Build history of the part. All positions in model axes, mm. A direction names the side the tool comes from. Give positions to 0.01 mm unless a question says otherwise; leave off trailing zeros. Loops run counter-clockwise (first coordinate to the right, second up) from the corner with the lowest first, then second, coordinate; pieces in that order, holes last. Notation, with made-up numbers: (8, 82) - (44, 82) arc R17 cw to (44, 88) - close; hole circle Ø9 at (5.25, 12.5). An arc over 180 degrees is marked (long way). Return JSON: item names as keys, results as strings. Group by question number.
1) Slice it at B-B (y = 46). List the corners of the cut face in (x, z), and give its area (3 significant figures).
2) Mould opens along Y. For faces 3 (the face through (-29.464, 25, 3)), 4 (the face through (-26, 47, 3.556)), 5 (the face through (-40.132, 25, 3)) say: released by +Y, released by -Y, zero draft, split by the parting line, or undercut.
3) Drill centre lines: probe 1 along X at (y, z) = (10.5, 2.6); probe 2 along Y at (x, z) = (-45, 2.8); probe 3 along X at (y, z) = (3.81, 2.65). Where is each one in solid material? Low to high. Write a range as from..to.
4) 3-axis set-ups, long thin cutter, end or side, ignore diameter. For faces 1 (the face through (-50.8, 25, 2)), 2 (the face through (-30.988, 25, 3)): which of +Z, -Z, +X, -X, +Y, -Y reach the whole face in a straight line?
5) Slice it at A-A (z = 2.7). Count the separate pieces of the cut face and the enclosed holes in it, and give its area (3 significant figures).
```python
from build123d import *

# Parameters (mm, degrees)
F0_W     = 50.8
F0_H     = 50.8
F1_DEPTH = 1.524
F2_W     = 50.8
F2_H     = 50.8
F2_W_2   = 46.736
F2_H_2   = 46.736
F2_W_3   = 43.688
F2_H_3   = 43.688
F2_W_4   = 39.624
F2_H_4   = 39.624
F2_W_5   = 36.576
F2_H_5   = 36.576
F2_W_6   = 32.512
F2_H_6   = 32.512
F2_W_7   = 29.464
F2_H_7   = 29.464
F2_W_8   = 25.4
F2_H_8   = 25.4
F2_W_9   = 22.352
F2_H_9   = 22.352
F2_W_10  = 18.288
F2_H_10  = 18.288
F2_W_11  = 15.24
F2_H_11  = 15.24
F2_W_12  = 11.176
F2_H_12  = 11.176
F2_W_13  = 8.128
F2_H_13  = 8.128
F3_DEPTH = 2.032
F4_R     = 1.4605
F5_DEPTH = 25.4


with BuildPart() as f1:
    # F0 (on Top) → F1 (new body)
    with BuildSketch(Plane.XY):
        with Locations((-25.4, 25.4)):
            Rectangle(F0_W, F0_H)
    extrude(amount=F1_DEPTH)

    # F2 (on face) → F3 (join)
    with BuildSketch(Plane.XY.offset(1.524)):
        with Locations((-25.4, 25.4)):
            Rectangle(F2_W, F2_H)
        with Locations((-25.4, 25.4)):
            Rectangle(F2_W_2, F2_H_2, mode=Mode.SUBTRACT)
        with Locations((-25.4, 25.4)):
            Rectangle(F2_W_3, F2_H_3)
        with Locations((-25.4, 25.4)):
            Rectangle(F2_W_4, F2_H_4, mode=Mode.SUBTRACT)
        with Locations((-25.4, 25.4)):
            Rectangle(F2_W_5, F2_H_5)
        with Locations((-25.4, 25.4)):
            Rectangle(F2_W_6, F2_H_6, mode=Mode.SUBTRACT)
        with Locations((-25.4, 25.4)):
            Rectangle(F2_W_7, F2_H_7)
        with Locations((-25.4, 25.4)):
            Rectangle(F2_W_8, F2_H_8, mode=Mode.SUBTRACT)
        with Locations((-25.4, 25.4)):
            Rectangle(F2_W_9, F2_H_9)
        with Locations((-25.4, 25.4)):
            Rectangle(F2_W_10, F2_H_10, mode=Mode.SUBTRACT)
        with Locations((-25.4, 25.4)):
            Rectangle(F2_W_11, F2_H_11)
        with Locations((-25.4, 25.4)):
            Rectangle(F2_W_12, F2_H_12, mode=Mode.SUBTRACT)
        with Locations((-25.4, 25.4)):
            Rectangle(F2_W_13, F2_H_13)
    extrude(amount=F3_DEPTH)

    # F4 (on face) → F5 (cut)
    with BuildSketch(Plane(origin=(0, 0, 0), x_dir=(1, 0, 0), z_dir=(0, 0, -1))):
        with Locations((-25.4, -3.81)):
            Circle(F4_R)
    extrude(amount=-F5_DEPTH, mode=Mode.SUBTRACT)


solid = f1.part
```
Results:
{
 "1": {"outline": "(-50.8, 0) - (0, 0) - (0, 3.56) - (-2.03, 3.56) - (-2.03, 1.52) - (-3.56, 1.52) - (-3.56, 3.56) - (-47.24, 3.56) - (-47.24, 1.52) - (-48.77, 1.52) - (-48.77, 3.56) - (-50.8, 3.56) - close", "area": "174 mm2"},
 "2": {"face 3": "undercut", "face 4": "zero draft", "face 5": "undercut"},
 "3": {"probe 1": "-50.8..-48.77, -47.24..-45.21, -43.69..-41.66, -9.14..-7.11, -5.59..-3.56, -2.03..0", "probe 2": "0..2.03, 3.56..5.59, 45.21..47.24, 48.77..50.8", "probe 3": "-50.8..-48.77, -47.24..-26.86, -23.94..-3.56, -2.03..0"},
 "4": {"face 1": "+Z, -Z, -X, +Y, -Y", "face 2": "+Z"},
 "5": {"separate pieces": "7", "enclosed holes": "6", "area": "1,570 mm2"}
}
